```python
from build123d import *

# Parameters (mm, degrees)
SKETCH_1_R      = 2
EXTRUDE_1_DEPTH = 30
SKETCH_2_R      = 3
EXTRUDE_2_DEPTH = 2
SKETCH_3_R      = 7.5
EXTRUDE_3_DEPTH = 14.5
FILLET_1_R      = 2
FILLET_2_R      = 0.5


with BuildPart() as part:
    # 草图1 → 凸台-拉伸1 (new body)
    with BuildSketch(Plane(origin=(0, 0, 0), x_dir=(1, 0, 0), z_dir=(0, 1, 0))):
        Circle(SKETCH_1_R)
    extrude(amount=EXTRUDE_1_DEPTH)

    # 草图2 → 凸台-拉伸2 (add)
    with BuildSketch(Plane(origin=(0, 30, 0), x_dir=(1, 0, 0), z_dir=(0, 1, 0))):
        Circle(SKETCH_2_R)
    extrude(amount=EXTRUDE_2_DEPTH)

    # 草图3 → 凸台-拉伸3 (add)
    with BuildSketch(Plane(origin=(0, 32, 0), x_dir=(1, 0, 0), z_dir=(0, 1, 0))):
        Circle(SKETCH_3_R)
    extrude(amount=EXTRUDE_3_DEPTH)

    # 圆角1
    fillet_1_edges = [part.edges().sort_by_distance(p)[0] for p in [
        (-7.5, 32, 0),
        (-7.5, 46.5, 0),
    ]]
    fillet(fillet_1_edges, radius=FILLET_1_R)

    # 圆角2
    fillet_2_edges = [part.edges().sort_by_distance(p)[0] for p in [
        (-3, 30, 0),
        (-3, 32, 0),
    ]]
    fillet(fillet_2_edges, radius=FILLET_2_R)


solid = part.part
```
Geometry check sheet. Reference: the model listing, model coordinates, mm. A direction names the side the tool comes from. Give positions to 0.01 mm unless a question says otherwise; leave off trailing zeros. Loops run counter-clockwise (first coordinate to the right, second up) from the corner with the lowest first, then second, coordinate; pieces in that order, holes last. Notation, with made-up numbers: M 35.25,63.5 L 67.25,63.5 A18 cw 67.25,94.5 Z; hole C 49.5,71.25 d8. An arc over 180 degrees is marked long. Answer as CSV lines item,"result".
Item 1: Cross-section at D-D on y = 27.5. Record the cut outline in (x, z), and give its area (3 significant figures).
Values:
outline,"C 0,0 d4"
area,"12.6 mm²"
Item 2: Cross-section at C-C on y = 38.5. Record the cut outline in (x, z), and give its area (3 significant figures).
Values:
outline,"C 0,0 d15"
area,"177 mm²"
Item 3: Cross-section at A-A on z = 0. Record the cut outline in (x, y), and give its area (3 significant figures).
Values:
outline,"M -7.5,34 A2 ccw -5.5,32 L -3.5,32 A0.5 cw -3,31.5 L -3,30.5 A0.5 ccw -2.5,30 L -2,30 L -2,0 L 2,0 L 2,30 L 2.5,30 A0.5 ccw 3,30.5 L 3,31.5 A0.5 cw 3.5,32 L 5.5,32 A2 ccw 7.5,34 L 7.5,44.5 A2 ccw 5.5,46.5 L -5.5,46.5 A2 ccw -7.5,44.5 Z"
area,"346 mm²"
Item 4: Material ranges on line 1 (Y direction, x = -4, z = 0.75); line 2 (Z direction, x = 5, y = 33.5); line 3 (Y direction, x = 0.5, z = 2.5), recorded low to high.
Values:
line 1,"y = 32 to 46.5"
line 2,"z = -5.5 to 5.5"
line 3,"y = 30 to 46.5"
Item 5: Depth check by flat-ended pin: P1, Ø5, axis at x = 3.5, z = 5.5, coming from the -Y side; P2, Ø1, axis at y = 19, z = -3.5, coming from the +X side; P3, Ø6, axis at x = 5.5, z = 0, coming from the -Y side. Enter the tip coordinate at first touch or a pass-through.
Values:
P1,"stops at y = 32"
P2,"passes through"
P3,"stops at y = 30"
Item 6: Cross-section at B-B on x = 0. Record the cut outline in (y, z), and give its area (3 significant figures).
Values:
outline,"M 0,-2 L 30,-2 L 30,-2.5 A0.5 ccw 30.5,-3 L 31.5,-3 A0.5 cw 32,-3.5 L 32,-5.5 A2 ccw 34,-7.5 L 44.5,-7.5 A2 ccw 46.5,-5.5 L 46.5,5.5 A2 ccw 44.5,7.5 L 34,7.5 A2 ccw 32,5.5 L 32,3.5 A0.5 cw 31.5,3 L 30.5,3 A0.5 ccw 30,2.5 L 30,2 L 0,2 Z"
area,"346 mm²"
Item 7: Access from +Z, -Z, +X, -X, +Y, -Y to the whole of each face (thin tool, end or side, straight path). Record for faces 1 (the cylindrical face through (0, 15, 2)), 2 (the flat face through (0, 46.5, 0)).
Values:
face 1,"-Y"
face 2,"+Z, -Z, +X, -X, +Y"
